Here's how the part is built. I have some questions about the finished solid (model axes, mm). A direction names the side the tool comes from. Coordinates: 2 decimals unless noted, no trailing zeros. Write each loop counter-clockwise with the first axis right and the second up, starting at its lowest first coordinate (ties: lowest second). Pieces come first, ordered by that corner, then holes.
Item 1: For faces 1 (the face through (18, 0, 0)), 2 (the face through (12.834, 0, 3)), 3 (the face through (12.768, -6.263, 3.234)), 4 (the face through (0, 0, 6.35)), 5 (the face through (0, 0, 0)), which set-ups out of +Z, -Z, +X, -X, +Y, -Y let a thin tool reach every point of the face, with its end or its side?
Item 2: If we mould it in two halves opening along Z, with no side actions, what happens to faces 6 (the face through (18.72, -10.35, 3.65)), 7 (the face through (17, 15.544, 3)), 8 (the face through (8.883, 0.768, 8.259))? For each: pulls with the +Z half, pulls with the -Z half, needs draft (parallel to the pull), parting line crosses it, or undercut.
Item 3: I want a section at D-D (y = 0). Please give me the cut outline in (x, z) (3 decimals), and give its area (3 significant figures).
Item 4: Please list where these lines run through material, in increasing order: line 1 (Z direction, x = 16.25, y = 0) (3 decimals); line 2 (X direction, y = -9.25, z = 5); line 3 (Z direction, x = 4, y = 1.75).
Item 5: I want a section at C-C (y = -9). Please give me the cut outline in (x, z).
Item 6: I want a section at A-A (z = 3). Please give me the cut outline in (x, y) (3 decimals).
Item 7: I'm going to push flat-ended pins straight in: P1, Ø3, axis at x = 1.5, y = 2.5, coming from the -Z side; P2, Ø6.5, axis at y = 12.5, z = 2, coming from the -X side; P3, Ø3, axis at y = -8.5, z = 3.5, coming from the -X side; P4, Ø1.2, axis at y = -9.44, z = 3.18, coming from the +X side. Where does each tip first touch, or does it pass through?
from build123d import *

# Parameters (mm, degrees)
BOSS_EXTRUDE1_DEPTH   = 6.35
BOSS_EXTRUDE2_START   = 3.175
BOSS_EXTRUDE2_DEPTH   = 12.7
CUT_EXTRUDE1_START    = -3.175
CUT_EXTRUDE1_DEPTH    = 6.35
F_1_CLEARANCE_HOLE1_D = 2.0574
FILLET4_START         = 4.487320853
FILLET4_DEPTH         = 18.252718486
FILLET5_R             = 5.08
CHAMFER3_SIZE         = 7.112
CHAMFER3_SIZE_2       = 3.316380065
BOSS_EXTRUDE3_START   = -7.9375
BOSS_EXTRUDE3_DEPTH   = 7.9375
F_1_CLEARANCE_HOLE2_D = 2.0574
SKETCH14_R            = 3.175
CUT_EXTRUDE2_DEPTH    = 27.974866065


with BuildPart() as part:
    # Sketch1 → Boss-Extrude1 (new body)
    with BuildSketch(Plane.XY):
        with BuildLine():
            Line((4.487320853, -2.38125), (4.487320853, 2.38125))
            ThreePointArc((4.487320853, 2.38125), (-5.08, 0), (4.487320853, -2.38125))
        make_face()
    extrude(amount=BOSS_EXTRUDE1_DEPTH)

    # Sketch2 → Boss-Extrude2 (add)
    with BuildSketch(Plane.XY.offset(6.35).offset(BOSS_EXTRUDE2_START)):
        Polygon((4.487320853, 2.38125), (4.487320853, -2.38125), (11.60035513, -7.606064703), (14.093661168, -9.4375), (22.740039339, -9.4375), (22.740039339, -7.631102389), (22.740039339, 7.631102389), (22.740039339, 15.543564703), (11.60035513, 15.543564703), (11.60035513, 7.606064703), align=None)
    extrude(amount=-BOSS_EXTRUDE2_DEPTH)

    # Sketch10 → Cut-Extrude1 (cut)
    with BuildSketch(Plane(origin=(0, 0, -3.175), x_dir=(-1, 0, 0), z_dir=(0, 0, -1)).offset(CUT_EXTRUDE1_START)):
        with BuildLine():
            Line((-22.740039339, -4.572), (-22.740039339, 4.572))
            ThreePointArc((-22.740039339, 4.572), (-22.329545252, 4.934830916), (-21.88930404, 5.260928055))
            Line((-21.88930404, 5.260928055), (-14.77730404, 5.260928055))
            ThreePointArc((-14.77730404, 5.260928055), (-13.687099855, 4.328427737), (-12.834042726, 3.175))
            Line((-12.834042726, 3.175), (-12.834042726, -3.175))
            ThreePointArc((-12.834042726, -3.175), (-13.687099855, -4.328427737), (-14.77730404, -5.260928055))
            Line((-14.77730404, -5.260928055), (-21.88930404, -5.260928055))
            ThreePointArc((-21.88930404, -5.260928055), (-22.329545252, -4.934830916), (-22.740039339, -4.572))
        make_face()
    extrude(amount=-CUT_EXTRUDE1_DEPTH, mode=Mode.SUBTRACT)

    # #1 Clearance Hole1 (through all)
    with Locations(Plane(origin=(22.740039339, 0, 0), x_dir=(0, 0, -1), z_dir=(1, 0, 0))):
        with Locations((-3.175, 9.4375)):
            Hole(F_1_CLEARANCE_HOLE1_D / 2)

    # Fillet4: read off the stored shape, not the designer's step
    # Fillet4 outline → Fillet4 (cut)
    with BuildSketch(Plane.YZ.offset(FILLET4_START)):
        with BuildLine():
            Line((-9.4375, -3.175), (-3.0875, -3.175))
            ThreePointArc((-3.0875, -3.175), (-7.577628061, -1.315128061), (-9.4375, 3.175))
            Line((-9.4375, 3.175), (-9.4375, -3.175))
        make_face()
        with BuildLine():
            Line((-9.4375, 9.525), (-9.4375, 3.175))
            ThreePointArc((-9.4375, 3.175), (-7.577628061, 7.665128061), (-3.0875, 9.525))
            Line((-3.0875, 9.525), (-9.4375, 9.525))
        make_face()
    extrude(amount=FILLET4_DEPTH, mode=Mode.SUBTRACT)

    # Fillet5
    fillet5_edges = [part.edges().sort_by_distance(p)[0] for p in [
        (17.170197235, 15.543564703, -3.175),
        (17.170197235, 15.543564703, 9.525),
    ]]
    fillet(fillet5_edges, radius=FILLET5_R)

    # Chamfer3
    # the kernel refuses this chamfer: 7.112, 3.316380065 mm, written as the material it takes off along each edge
    with BuildSketch(Plane(origin=(4.487320853, 20.808267553, -3.175), x_dir=(1, 0, 0), z_dir=(0, -1, 0))) as chamfer3_piece_1_section:
        Polygon((CHAMFER3_SIZE, 0), (0, CHAMFER3_SIZE_2), (0, 0), align=None)
    chamfer3_piece_1 = extrude(amount=41.616535106, mode=Mode.PRIVATE)
    chamfer3_piece_1 = chamfer3_piece_1 - Plane(origin=(0, 0, -3.175), x_dir=(0.8833308765689106, 0.46875000000000017, 0), z_dir=(0, 0, -1)) * Cylinder(5.08, 112, mode=Mode.PRIVATE)
    add(chamfer3_piece_1, mode=Mode.SUBTRACT)
    with BuildSketch(Plane(origin=(4.487320853, 20.808267553, -3.175), x_dir=(1, 0, 0), z_dir=(0, -1, 0))) as chamfer3_piece_2_section:
        Polygon((CHAMFER3_SIZE, 0), (0, CHAMFER3_SIZE_2), (0, 0), align=None)
    chamfer3_piece_2 = extrude(amount=41.616535106, mode=Mode.PRIVATE)
    chamfer3_piece_2 = split(chamfer3_piece_2, bisect_by=Plane(origin=(4.487320853, 20.808267553, 0), z_dir=(0, 0, -1)), keep=Keep.TOP, mode=Mode.PRIVATE)
    add(chamfer3_piece_2, mode=Mode.SUBTRACT)
    with BuildSketch(Plane(origin=(4.487320853, 20.808267553, 9.525), x_dir=(1, 0, 0), z_dir=(0, -1, 0))) as chamfer3_piece_3_section:
        Polygon((CHAMFER3_SIZE, 0), (0, -CHAMFER3_SIZE_2), (0, 0), align=None)
    chamfer3_piece_3 = extrude(amount=41.616535106, mode=Mode.PRIVATE)
    chamfer3_piece_3 = chamfer3_piece_3 - Plane(origin=(0, 0, 9.525), x_dir=(0.8833308765689106, 0.46875000000000017, 0), z_dir=(0, 0, -1)) * Cylinder(5.08, 112, mode=Mode.PRIVATE)
    add(chamfer3_piece_3, mode=Mode.SUBTRACT)
    with BuildSketch(Plane(origin=(4.487320853, 20.808267553, 9.525), x_dir=(1, 0, 0), z_dir=(0, -1, 0))) as chamfer3_piece_4_section:
        Polygon((CHAMFER3_SIZE, 0), (0, -CHAMFER3_SIZE_2), (0, 0), align=None)
    chamfer3_piece_4 = extrude(amount=41.616535106, mode=Mode.PRIVATE)
    chamfer3_piece_4 = split(chamfer3_piece_4, bisect_by=Plane(origin=(4.487320853, 20.808267553, 6.35), z_dir=(0, 0, 1)), keep=Keep.TOP, mode=Mode.PRIVATE)
    add(chamfer3_piece_4, mode=Mode.SUBTRACT)

    # Sketch11 → Boss-Extrude3 (add)
    with BuildSketch(Plane(origin=(22.740039339, 0, 0), x_dir=(0, 0, -1), z_dir=(1, 0, 0)).offset(BOSS_EXTRUDE3_START)):
        with BuildLine():
            ThreePointArc((-6.249180531, -8.64375), (-3.175, -12.6125), (-0.100819469, -8.64375))
            ThreePointArc((-0.100819469, -8.64375), (-3.175, -9.4375), (-6.249180531, -8.64375))
        make_face()
    extrude(amount=BOSS_EXTRUDE3_DEPTH)

    # #1 Clearance Hole2 (through all)
    with Locations(Plane(origin=(22.740039339, 0, 0), x_dir=(0, 0, -1), z_dir=(1, 0, 0))):
        with Locations((-3.175, -9.4375)):
            Hole(F_1_CLEARANCE_HOLE2_D / 2)

    # Sketch14 → Cut-Extrude2 (cut, through all)
    with BuildSketch(Plane.ZY.offset(-14.802539339)):
        with Locations((3.175, -9.4375)):
            Circle(SKETCH14_R)
    extrude(amount=CUT_EXTRUDE2_DEPTH, mode=Mode.SUBTRACT)


solid = part.part
Answer:
1. face 1: none
1. face 2: +X
1. face 3: -X, -Y
1. face 4: +Z, -X, +Y, -Y
1. face 5: -Z, -X, +Y, -Y
2. face 6: undercut
2. face 7: needs draft
2. face 8: pulls with the +Z half
3. outline: (-5.08, 0) - (4.791, 0) - (11.599, -3.175) - (22.74, -3.175) - (22.74, 0) - (12.834, 0) - (12.834, 6.35) - (22.74, 6.35) - (22.74, 9.525) - (11.599, 9.525) - (4.791, 6.35) - (-5.08, 6.35) - close
3. area: 206 mm2
4. line 1: z = -3.175 to 0, 6.35 to 9.525
4. line 2: x = 14.8 to 22.74
4. line 3: z = 0 to 6.35
5. outline: (14.8, 0.03) - (22.74, 0.03) - (22.74, 2.24) - (14.8, 2.24) - close; (14.8, 4.11) - (22.74, 4.11) - (22.74, 6.32) - (14.8, 6.32) - close
6. outline: (4.487, -2.381) - (9.778, -6.267) - (14.803, -6.267) - (14.803, -8.424) - (22.74, -8.424) - (22.74, -4.572) arc R6.35 cw to (21.889, -5.261) - (14.777, -5.261) arc R6.35 cw to (12.834, -3.175) - (12.834, 3.175) arc R6.35 cw to (14.777, 5.261) - (21.889, 5.261) arc R6.35 cw to (22.74, 4.572) - (22.74, 8.424) - (11.6, 8.424) - (11.6, 7.606) - (4.487, 2.381) arc R5.08 ccw (long way) to start; (11.6, 10.451) - (22.74, 10.451) - (22.74, 15.544) - (11.6, 15.544) - close; (14.803, -12.608) - (22.74, -12.608) - (22.74, -10.451) - (14.803, -10.451) - close
7. P1: stops at z = 0
7. P2: stops at x = 11.6
7. P3: stops at x = 14.8
7. P4: passes through
